from build123d import *

# Parameters (mm, degrees)
MODEL_R             = 1.5
BOSS_EXTRUDE1_DEPTH = 6.6


with BuildPart() as part:
    # Model → Boss-Extrude1 (new body)
    with BuildSketch(Plane.XY):
        with BuildLine():
            Line((0.403470192, -13.809994881), (-2.071067812, -13.4))
            ThreePointArc((-2.071067812, -13.4), (-4.374720312, -11.399768226), (-5.087238474, -8.433278742))
            ThreePointArc((-5.087238474, -8.433278742), (-4.773776994, 0), (-5.087238474, 8.433278742))
            ThreePointArc((-5.087238474, 8.433278742), (-4.374720312, 11.399768226), (-2.071067812, 13.4))
            Line((-2.071067812, 13.4), (0.403470192, 13.809994881))
            ThreePointArc((0.403470192, 13.809994881), (4.346933521, 17.214586867), (3.121718942, 22.278281058))
            Line((3.121718942, 22.278281058), (1.464466094, 23.935533906))
            ThreePointArc((1.464466094, 23.935533906), (-0.15765065, 25.019397663), (-2.071067812, 25.4))
            Line((-2.071067812, 25.4), (-13.74395333, 25.4))
            ThreePointArc((-13.74395333, 25.4), (-17.602984306, 23.579289217), (-18.651543558, 19.44315197))
            ThreePointArc((-18.651543558, 19.44315197), (-16.773776994, 0), (-18.651543558, -19.44315197))
            ThreePointArc((-18.651543558, -19.44315197), (-17.602984306, -23.579289217), (-13.74395333, -25.4))
            Line((-13.74395333, -25.4), (-2.071067812, -25.4))
            ThreePointArc((-2.071067812, -25.4), (-0.15765065, -25.019397663), (1.464466094, -23.935533906))
            Line((1.464466094, -23.935533906), (3.121718942, -22.278281058))
            ThreePointArc((3.121718942, -22.278281058), (4.346933521, -17.214586867), (0.403470192, -13.809994881))
        make_face()
        with Locations((0.325033172, 18.5)):
            Circle(MODEL_R, mode=Mode.SUBTRACT)
        with Locations((0.348456442, -18.5)):
            Circle(MODEL_R, mode=Mode.SUBTRACT)
    extrude(amount=BOSS_EXTRUDE1_DEPTH)


solid = part.part
The model under review builds one solid part; all positions refer to its coordinate system, in mm. A direction names the side the tool comes from. Coordinates: 2 decimals unless noted, no trailing zeros. Loops run counter-clockwise (first coordinate to the right, second up) from the corner with the lowest first, then second, coordinate; pieces in that order, holes last.
(1) Tool access review of faces 1 (the flat face through (-0.816, -13.608, 3.254)), 2 (the cylindrical face through (-0.13, 25.01, 3.25)): name each direction out of +Z, -Z, +X, -X, +Y, -Y from which nothing blocks a thin tool from reaching the whole face with its end or side.
Determined:
face 1: +Z, -Z, +X
face 2: +Z, -Z, +X, +Y
(2) Draft analysis for pull direction Y (two halves, no side actions). For faces 3 (the cylindrical face through (0.13, 19.987, 3.254)), 4 (the flat face through (2.3, 23.1, 3.3)), 5 (the flat face through (-10, 0, 0)), state which applies: +Y half, -Y half, draft (parallel to the pull), parting line (faces both ways), or undercut.
Determined:
face 3: undercut
face 4: +Y half
face 5: draft
(3) Consider section C-C, the plane y = 6.5. Give the boundary of the cut face in (x, z).
Determined:
outline: (-16.98, 0) - (-4.96, 0) - (-4.96, 6.6) - (-16.98, 6.6) - close
(4) Wall thickness on L1, parallel to Y at x = 2.25, z = 1; L2, parallel to X at y = 8.5, z = 2.25; L3, parallel to Y at x = -3.25, z = 3: over which ranges is each line inside the solid? List them lowest first.
Determined:
L1: y = -23.15 to -14.51, 14.51 to 23.15
L2: x = -17.13 to -5.09
L3: y = -25.4 to -12.69, 12.69 to 25.4
(5) Insertion check: P1, Ø3, axis at y = -17, z = 5, coming from the +X side; P2, Ø3, axis at x = -16, z = 0.5, coming from the -Y side; P3, Ø2, axis at y = 12, z = 3.5, coming from the -X side; P4, Ø2.5, axis at x = 0.33, y = 18.5, coming from the -Z side. Each pin has a flat end and moves straight along its axis. Give the tip position at first contact, or say it passes through.
Determined:
P1: stops at x = 4.58
P2: stops at y = -25.34
P3: stops at x = -17.61
P4: passes through
(6) Consider section A-A, the plane z = 2.5. Give the boundary of the cut face in (x, y).
Determined:
outline: (-18.65, -19.44) arc R5 ccw to (-13.74, -25.4) - (-2.07, -25.4) arc R5 ccw to (1.46, -23.94) - (3.12, -22.28) arc R5 ccw to (0.4, -13.81) - (-2.07, -13.4) arc R5 cw to (-5.09, -8.43) arc R113.6 ccw to (-5.09, 8.43) arc R5 cw to (-2.07, 13.4) - (0.4, 13.81) arc R5 ccw to (3.12, 22.28) - (1.46, 23.94) arc R5 ccw to (-2.07, 25.4) - (-13.74, 25.4) arc R5 ccw to (-18.65, 19.44) arc R101.6 cw to start; hole circle Ø3 at (0.33, 18.5); hole circle Ø3 at (0.35, -18.5)
(7) Consider section B-B, the plane y = -18.5. Give the boundary of the cut face in (x, z).
Determined:
outline: (-18.47, 0) - (-1.15, 0) - (-1.15, 6.6) - (-18.47, 6.6) - close; (1.85, 0) - (4.58, 0) - (4.58, 6.6) - (1.85, 6.6) - close
